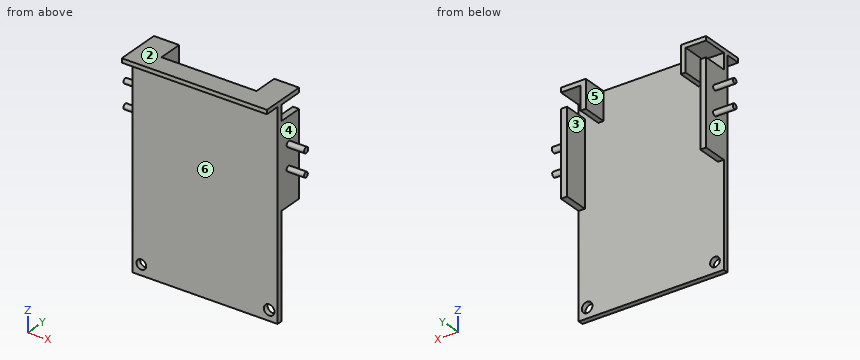
```python
from build123d import *

# Parameters (mm, degrees)
F0_W     = 88.9
F0_H     = 127
F0_R     = 2.9848451786
F0_R_2   = 3.2536679358
F1_DEPTH = 3.175
F2_W     = 88.9
F2_H     = 2.54
F3_DEPTH = 9.14618
F4_W     = 3.1831779712
F4_H     = 14.4224017859
F4_W_2   = 3.8154479831
F4_H_2   = 51.5085849911
F4_W_3   = 2.9760506004
F4_H_3   = 14.1934752464
F4_W_4   = 3.5865214437
F4_H_4   = 51.7375124618
F5_DEPTH = 15.11912
F6_R     = 1.7434569234
F6_R_2   = 1.6024885699
F7_DEPTH = 10.69614
F8_R     = 1.5356896605
F8_R_2   = 1.6187597598
F9_DEPTH = 12.03988


with BuildPart() as f1:
    # F0 (on Front) → F1 (new body)
    with BuildSketch(Plane.XZ):
        with Locations((-0.1144651324, -7.7015060779)):
            Rectangle(F0_W, F0_H)
        with Locations((-39.1465239227, -64.9008154869)):
            Circle(F0_R, mode=Mode.SUBTRACT)
        with Locations((39.1465201974, -64.9008154869)):
            Circle(F0_R_2, mode=Mode.SUBTRACT)
    extrude(amount=F1_DEPTH)

    # F2 (on face) → F3 (join)
    with BuildSketch(Plane.XZ.offset(3.175)):
        with Locations((-0.1144651324, 54.5284939221)):
            Rectangle(F2_W, F2_H)
    extrude(amount=F3_DEPTH)

    # F4 (on face) → F5 (join)
    with BuildSketch(Plane(origin=(0, 0, 0), x_dir=(-1, 0, 0), z_dir=(0, 1, 0))):
        Polygon((-29.0955348676, 55.4166970754), (-29.0955348676, 55.7984939221), (-44.3355348676, 55.7984939221), (-44.3355348676, 55.4166970754), (-44.3355348676, 52.99660936), (-32.2787128389, 52.99660936), (-29.0955348676, 52.99660936), align=None)
        with Locations((-30.6871238533, 45.7854084671)):
            Rectangle(F4_W, F4_H)
        with Locations((-42.4278108761, 17.8563101217)):
            Rectangle(F4_W_2, F4_H_2)
        Polygon((44.5644651324, 55.7984939221), (29.0737356991, 55.7984939221), (29.0737356991, 53.2255358994), (32.0497862995, 53.2255358994), (40.7490134239, 53.2255358994), (44.5644651324, 53.2255358994), align=None)
        with Locations((30.5617609993, 46.1287982762)):
            Rectangle(F4_W_3, F4_H_3)
        with Locations((42.7712044105, 17.7418463863)):
            Rectangle(F4_W_4, F4_H_4)
    extrude(amount=F5_DEPTH)

    # F6 (on face) → F7 (join)
    with BuildSketch(Plane.YZ.offset(44.3355348676)):
        with Locations((6.2954924069, 27.5857094675)):
            Circle(F6_R)
        with Locations((6.0665672645, 13.6211588979)):
            Circle(F6_R_2)
    extrude(amount=F7_DEPTH)

    # F8 (on face) → F9 (join)
    with BuildSketch(Plane(origin=(-44.5644651324, 0, 0), x_dir=(0, -1, 0), z_dir=(-1, 0, 0))):
        with Locations((-7.554592099, 29.6460520476)):
            Circle(F8_R)
        with Locations((-7.554592099, 14.9947218597)):
            Circle(F8_R_2)
    extrude(amount=F9_DEPTH)


solid = f1.part
```
Read the model definition and answer for the solid it produces. Units are mm, in the model's axes. Face numbers are marked on the shaded views. A direction names the side the tool comes from. Coordinates: 2 decimals unless noted, no trailing zeros. Order: outer loops, then holes, each group sorted by start corner. A loop starts at its lowest first (then second) coordinate and runs counter-clockwise, first axis right, second up. Notation, with made-up numbers: (-30, 13.5) - (23, 13.5) arc R10 ccw to (23, 29.5) - close; hole circle Ø8 at (-33.5, 43.25). An arc over 180 degrees is marked (long way). Answer as a JSON object with one key per item and string values. Group by question number.
Item 1: Section B-B (z = 33) is taken. Give the vertices of the cut face in (x, y) (3 decimals), plus the area to 3 significant figures.
Item 2: The mould has two halves that part along X. Classify the marked faces 1, 2, 3 and 4: +X half, -X half, draft (parallel to the pull), parting line (faces both ways), or undercut.
Item 3: Section D-D (z = 46) is taken. Give the vertices of the cut face in (x, y) (3 decimals), plus the area to 3 significant figures.
Item 4: Consider probe 1 along X at (y, z) = (4.5, 41); probe 2 along X at (y, z) = (2.25, 45.5); probe 3 along Z at (x, y) = (43, 7). Determine where each line is inside the solid, lowest interval first. Write a range as from..to.
Item 5: Flat-ended cylindrical pins translate along their axes: P1, Ø1, axis at y = 8, z = -3, coming from the -X side; P2, Ø1.5, axis at x = 36.5, y = 1.5, coming from the -Z side; P3, Ø1.1, axis at x = 43, y = 10, coming from the -Z side. Find the tip coordinate at first contact, or state that the pin passes through.
Item 6: Section C-C (x = 27) is taken. Give the vertices of the cut face in (y, z) (1 decimal).
Item 7: Section A-A (y = 13.5) is taken. Give the vertices of the cut face in (x, z), plus the area to 3 significant figures.
Item 8: A tool of negligible diameter and unlimited length cuts with its end or side. For the marked faces 5 and 6, from which of +Z, -Z, +X, -X, +Y, -Y can it reach the whole face along a straight path? Write none if from no direction.
Results are:
{
 "1": {"outline": "(-44.564, -3.175) - (44.336, -3.175) - (44.336, 15.119) - (40.52, 15.119) - (40.52, 0) - (-40.978, 0) - (-40.978, 15.119) - (-44.564, 15.119) - close", "area": "394 mm^2"},
 "2": {"face 1": "-X half", "face 2": "draft", "face 3": "undercut", "face 4": "+X half"},
 "3": {"outline": "(-44.564, -3.175) - (44.336, -3.175) - (44.336, 0) - (32.279, 0) - (32.279, 15.119) - (29.096, 15.119) - (29.096, 0) - (-29.074, 0) - (-29.074, 15.119) - (-32.05, 15.119) - (-32.05, 0) - (-44.564, 0) - close", "area": "375 mm^2"},
 "4": {"probe 1": "x = -44.56..-40.98, -32.05..-29.07, 29.1..32.28, 40.52..44.34", "probe 2": "x = -32.05..-29.07, 29.1..32.28", "probe 3": "z = -7.9..43.61, 53..55.8"},
 "5": {"P1": "stops at x = -44.56", "P2": "stops at z = 53", "P3": "stops at z = -7.9"},
 "6": {"outline": "(-12.3, 53.3) - (-3.2, 53.3) - (-3.2, -71.2) - (0, -71.2) - (0, 55.8) - (-12.3, 55.8) - close"},
 "7": {"outline": "(-44.56, -8.13) - (-40.98, -8.13) - (-40.98, 43.61) - (-44.56, 43.61) - close; (-44.56, 53.23) - (-32.05, 53.23) - (-32.05, 39.03) - (-29.07, 39.03) - (-29.07, 55.8) - (-44.56, 55.8) - close; (29.1, 38.57) - (32.28, 38.57) - (32.28, 53) - (44.34, 53) - (44.34, 55.8) - (29.1, 55.8) - close; (40.52, -7.9) - (44.34, -7.9) - (44.34, 43.61) - (40.52, 43.61) - close", "area": "553 mm^2"},
 "8": {"face 5": "+Z, -Z, +Y", "face 6": "-Z, +X, -X, -Y"}
}
